Verification items for the finished model (mm, model axes). Coordinates: 2 decimals unless noted, no trailing zeros. Write each loop counter-clockwise with the first axis right and the second up, starting at its lowest first coordinate (ties: lowest second). Pieces come first, ordered by that corner, then holes. Notation, with made-up numbers: (-34.5, 29.25) -> (-14.5, 29.25) arc R10 cw to (-14.5, 37.25) -> close; hole circle Ø5 at (-7, 17.25). An arc over 180 degrees is marked (long way). Answer in a Markdown table with one row per item.
```python
from build123d import *

# Parameters (mm, degrees)
BOSS_EXTRU_1_DEPTH      = 6
ENL_V_MAT_EXTRU_1_REACH = 8
ESQUISSE2_R             = 2.5


with BuildPart() as part:
    # Esquisse1 → Boss.-Extru.1 (new body)
    with BuildSketch(Plane.XY):
        Polygon((0, 5.773502692), (-5, 2.886751346), (-5, -2.886751346), (0, -5.773502692), (5, -2.886751346), (5, 2.886751346), align=None)
    extrude(amount=BOSS_EXTRU_1_DEPTH)

    # Esquisse2 → Enlèv. mat.-Extru.1 (cut, up to next)
    with BuildSketch(Plane.XY.offset(6), mode=Mode.PRIVATE) as enl_v_mat_extru_1_sk1:
        Circle(ESQUISSE2_R)
    enl_v_mat_extru_1_tool1 = extrude(enl_v_mat_extru_1_sk1.sketch, amount=-ENL_V_MAT_EXTRU_1_REACH, mode=Mode.PRIVATE) & part.part
    add(enl_v_mat_extru_1_tool1.solids().sort_by_distance((0, 0, 6))[0], mode=Mode.SUBTRACT)

    # Esquisse4 → Enlèvement de matière-Révolution8 (revolve, cut)
    with BuildSketch(Plane(origin=(0, 0, 0), x_dir=(1, 0, 0), z_dir=(0, 1, 0))):
        Polygon((-10.196152423, -3), (-3.267949192, 1), (-11.196152423, 1), (-11.196152423, -7), (-3.267949192, -7), align=None)
    revolve(axis=Axis((0, 0, 0), (0, 0, 1)), mode=Mode.SUBTRACT)


solid = part.part
```
1. Mould release check, pull along X, two halves, no side actions. Record for faces 1 (the conical face through (4.49, -2.6, 5.89)), 2 (the flat face through (-5, 0, 3)), 3 (the flat face through (2, -2, 0)), 4 (the cylindrical face through (-0.54, -2.44, 3.04)): released by +X, released by -X, zero draft, split by the parting line, or undercut.
Geometry says:
| item | result |
|---|---|
| face 1 | released by +X |
| face 2 | released by -X |
| face 3 | zero draft |
| face 4 | undercut |
2. Section check A-A, the plane z = 1.05. Record the boundary of the cut face in (x, y).
Geometry says:
| item | result |
|---|---|
| outline | (-5, -2.89) -> (0, -5.77) -> (5, -2.89) -> (5, 2.89) -> (0, 5.77) -> (-5, 2.89) -> close; hole circle Ø5 at (0, 0) |
3. Thickness scan on line 1 (X direction, y = -0.75, z = 2.75); line 2 (X direction, y = 2, z = 2.85); line 3 (Y direction, x = 4.25, z = 2.35). Record the ranges inside material, lowest first. Write a range as from..to.
Geometry says:
| item | result |
|---|---|
| line 1 | -5..-2.38, 2.38..5 |
| line 2 | -5..-1.5, 1.5..5 |
| line 3 | -3.32..3.32 |
